Read the model definition and answer for the solid it produces. Units are mm, in the model's axes. A direction names the side the tool comes from. Coordinates: 2 decimals unless noted, no trailing zeros. Write each loop counter-clockwise with the first axis right and the second up, starting at its lowest first coordinate (ties: lowest second). Pieces come first, ordered by that corner, then holes. Notation, with made-up numbers: (25.25, -21.5) -> (64.25, -21.5) arc R32 cw to (64.25, 17.5) -> close; hole circle Ø5 at (65, -6). An arc over 180 degrees is marked (long way). Write item = value, one per line. Start each with the question number.
1) Find the intervals of material crossed by line 1 along Y through (x, z) = (0, 1); line 2 along Y through (x, z) = (-0.5, 5.5); line 3 along Y through (x, z) = (-1, 8.75), in increasing order. Write a range as from..to.
2) Section A-A (x = 0) is taken. Determine the outline of the cut face in (y, z), plus the area to 3 significant figures.
3) Section C-C (y = -1.75) is taken. Determine the outline of the cut face in (x, z).
4) A flat-ended cylindrical pin translates along its axis: pin 1 Ø3.5 at (x, y) = (-2, 0.5) entering from +Z. Find the tip coordinate at first contact, or state that the pin passes through.
5) A tool of negligible diameter and unlimited length cuts with its end or side. For faces 5 (the face through (-0.3, -8, 8.5)), 6 (the face through (-3.17, 1.87, 6.03)), 7 (the face through (0, -9, 9)), from which of +Z, -Z, +X, -X, +Y, -Y can it reach the whole face along a straight path? Write none if from no direction.
6) For a pull along X with two mould halves and no side action, classify faces 1 (the face through (-0.3, 2.4, 0)), 2 (the face through (-25, 0, 4)), 3 (the face through (3.17, -1.87, 6.03)), 4 (the face through (25, 0, 4)) as released by +X, released by -X, zero draft, split by the parting line, or undercut.
7) Section B-B (z = 1.25) is taken. Determine the outline of the cut face in (x, y), plus the area to 3 significant figures.
8) Section D-D (z = 7.25) is taken. Determine the outline of the cut face in (x, y) (3 decimals), plus the area to 3 significant figures.
from build123d import *

# Parameters (mm, degrees)
SKETCH_W        = 50
SKETCH_H        = 20
PAD_DEPTH       = 9
SKETCH001_R     = 2.25
POCKET_DEPTH    = 9
POCKET001_DEPTH = 5
SKETCH003_W     = 50
SKETCH003_H     = 18
POCKET002_DEPTH = 1


with BuildPart() as part:
    # Sketch → Pad (new body)
    with BuildSketch(Plane.XY):
        Rectangle(SKETCH_W, SKETCH_H)
    extrude(amount=PAD_DEPTH)

    # Sketch001 (on DatumPlane) → Pocket (cut)
    with BuildSketch(Plane.XY.offset(9)):
        Circle(SKETCH001_R)
    extrude(amount=-POCKET_DEPTH, mode=Mode.SUBTRACT)

    # Sketch002 (on DatumPlane) → Pocket001 (cut)
    with BuildSketch(Plane.XY.offset(9)):
        Polygon((2.125, -3.680608), (4.25, 0), (2.125, 3.680608), (-2.125, 3.680608), (-4.25, 0), (-2.125, -3.680608), align=None)
    extrude(amount=-POCKET001_DEPTH, mode=Mode.SUBTRACT)

    # Sketch003 (on DatumPlane) → Pocket002 (cut)
    with BuildSketch(Plane.XY.offset(9)):
        with Locations((0, 1)):
            Rectangle(SKETCH003_W, SKETCH003_H)
    extrude(amount=-POCKET002_DEPTH, mode=Mode.SUBTRACT)


solid = part.part
Answer key:
q1.line_1 = -10..-2.25, 2.25..10
q1.line_2 = -10..-3.68, 3.68..10
q1.line_3 = -10..-8
q2.outline = (-10, 0) -> (-2.25, 0) -> (-2.25, 4) -> (-3.68, 4) -> (-3.68, 8) -> (-8, 8) -> (-8, 9) -> (-10, 9) -> close; (2.25, 0) -> (10, 0) -> (10, 8) -> (3.68, 8) -> (3.68, 4) -> (2.25, 4) -> close
q2.area = 115 mm^2
q3.outline = (-25, 0) -> (-1.41, 0) -> (-1.41, 4) -> (-3.24, 4) -> (-3.24, 8) -> (-25, 8) -> close; (1.41, 0) -> (25, 0) -> (25, 8) -> (3.24, 8) -> (3.24, 4) -> (1.41, 4) -> close
q4.pin_1 = 8
q5.face_5 = +Z, +X, -X, +Y
q5.face_6 = +Z
q5.face_7 = +Z, +X, -X, +Y, -Y
q6.face_1 = zero draft
q6.face_2 = released by -X
q6.face_3 = undercut
q6.face_4 = released by +X
q7.outline = (-25, -10) -> (25, -10) -> (25, 10) -> (-25, 10) -> close; hole circle Ø4.5 at (0, 0)
q7.area = 984 mm^2
q8.outline = (-25, -10) -> (25, -10) -> (25, 10) -> (-25, 10) -> close; hole (-4.25, 0) -> (-2.125, -3.681) -> (2.125, -3.681) -> (4.25, 0) -> (2.125, 3.681) -> (-2.125, 3.681) -> close
q8.area = 953 mm^2
